The model under review builds one solid part; all positions refer to its coordinate system, in mm. Face numbers are marked on the shaded views. A direction names the side the tool comes from. Give positions to 0.01 mm unless a question says otherwise; leave off trailing zeros. Order: outer loops, then holes, each group sorted by start corner. A loop starts at its lowest first (then second) coordinate and runs counter-clockwise, first axis right, second up. Notation, with made-up numbers: (-20.75, 57.25) -> (-0.75, 57.25) arc R29 cw to (-0.75, 82.25) -> close; hole circle Ø9 at (27, 36.5). An arc over 180 degrees is marked (long way). Use one line per item in the form item = value.
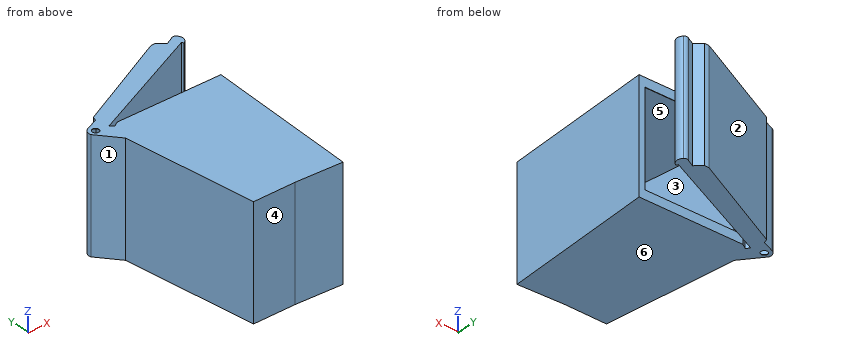
```python
from build123d import *

# Parameters (mm, degrees)
BOSS_EXTRUDE1_DEPTH = 6.35
SHELL1_START        = 0.0254
SHELL1_DEPTH        = 6.2992
SKETCH3_W           = 5.418512696
SKETCH3_H           = 5.334
CUT_EXTRUDE2_DEPTH  = 1.524
SKETCH4_R           = 0.1905
CUT_EXTRUDE3_DEPTH  = 20.633989303


# Read off the part's stored shape, not the designer's step: Shell1
with BuildPart() as part:
    # Sketch1 → Boss-Extrude1 (new body)
    with BuildSketch(Plane.XY):
        with BuildLine():
            Line((7.716040042, 1.833305163), (10.375382868, 1.693751976))
            Line((10.375382868, 1.693751976), (11.029172055, 10.583751976))
            Line((11.029172055, 10.583751976), (5.064666493, 10.656097731))
            Line((5.064666493, 10.656097731), (4.767245057, 10.479252552))
            Line((4.767245057, 10.479252552), (4.590399878, 10.656097731))
            Line((4.590399878, 10.656097731), (11.46006589, 13.704368441))
            Line((11.46006589, 13.704368441), (11.509343406, 13.593315288))
            ThreePointArc((11.509343406, 13.593315288), (11.739536715, 13.882052013), (11.634947175, 14.236197299))
            ThreePointArc((11.634947175, 14.236197299), (11.492158572, 14.298396741), (11.347210136, 14.241411598))
            Line((11.347210136, 14.241411598), (10.931187512, 14.042030874))
            Line((10.931187512, 14.042030874), (10.548202312, 14.393751976))
            Line((10.548202312, 14.393751976), (10.290273504, 14.393751976))
            Line((10.290273504, 14.393751976), (4.530564215, 11.633385245))
            Line((4.530564215, 11.633385245), (4.445957531, 11.39304745))
            Line((4.445957531, 11.39304745), (3.74568803, 11.102479142))
            ThreePointArc((3.74568803, 11.102479142), (3.54655055, 10.911956466), (3.527947792, 10.636986353))
            Line((3.527947792, 10.636986353), (4.481389231, 9.429510304))
            Line((4.481389231, 9.429510304), (5.295382868, 1.833305163))
            Line((5.295382868, 1.833305163), (7.716040042, 1.833305163))
        make_face()
    extrude(amount=BOSS_EXTRUDE1_DEPTH)

    # Shell1 outline → Shell1 (cut)
    with BuildSketch(Plane.XY.offset(SHELL1_START)):
        with BuildLine():
            Line((5.318206472, 1.858705163), (7.716706036, 1.858705163))
            Line((7.716706036, 1.858705163), (10.351875533, 1.720420509))
            Line((10.351875533, 1.720420509), (11.001859717, 10.558681389))
            Line((11.001859717, 10.558681389), (5.071504797, 10.630612918))
            Line((5.071504797, 10.630612918), (4.76325019, 10.447326395))
            Line((4.76325019, 10.447326395), (4.546271575, 10.664305009))
            Line((4.546271575, 10.664305009), (11.472980817, 13.737887461))
            Line((11.472980817, 13.737887461), (11.521908422, 13.627622875))
            ThreePointArc((11.521908422, 13.627622875), (11.716832945, 13.899435369), (11.616664188, 14.218565158))
            ThreePointArc((11.616664188, 14.218565158), (11.489713166, 14.273025818), (11.362015112, 14.220340596))
            Line((11.362015112, 14.220340596), (10.926665769, 14.011697454))
            Line((10.926665769, 14.011697454), (10.538308623, 14.368351976))
            Line((10.538308623, 14.368351976), (10.296045707, 14.368351976))
            Line((10.296045707, 14.368351976), (4.551029407, 11.615026927))
            Line((4.551029407, 11.615026927), (4.466154882, 11.373928288))
            Line((4.466154882, 11.373928288), (3.755422691, 11.079018614))
            ThreePointArc((3.755422691, 11.079018614), (3.570543876, 10.903284548), (3.550847191, 10.64897238))
            Line((3.550847191, 10.64897238), (4.505864047, 9.439501161))
            Line((4.505864047, 9.439501161), (5.318206472, 1.858705163))
        make_face()
    extrude(amount=SHELL1_DEPTH, mode=Mode.SUBTRACT)

    # Sketch3 → Cut-Extrude2 (cut)
    with BuildSketch(Plane(origin=(0.12997786, 10.715952445, 0), x_dir=(0.9999264471855748, -0.012128487903857954, 0), z_dir=(0.012128487903857952, 0.9999264471855747, 0))):
        with Locations((7.850713163, -3.175)):
            Rectangle(SKETCH3_W, SKETCH3_H)
    extrude(amount=-CUT_EXTRUDE2_DEPTH, mode=Mode.SUBTRACT)

    # Sketch4 → Cut-Extrude3 (cut, through all)
    with BuildSketch(Plane.XY.offset(6.35)):
        with Locations((3.89174221, 10.750488628)):
            Circle(SKETCH4_R)
    extrude(amount=-CUT_EXTRUDE3_DEPTH, mode=Mode.SUBTRACT)


solid = part.part
```
1. Add section B-B on y = 3.5. Give the boundary of the cut face in (x, z), then the cut area to 3 significant figures.
Values:
outline = (5.12, 0) -> (10.51, 0) -> (10.51, 6.35) -> (5.12, 6.35) -> close; hole (5.14, 0.03) -> (10.48, 0.03) -> (10.48, 6.32) -> (5.14, 6.32) -> close
area = 0.595 mm^2
2. Tool access review of the marked faces 4, 5 and 6: name each direction out of +Z, -Z, +X, -X, +Y, -Y from which nothing blocks a thin tool from reaching the whole face with its end or side.
Values:
face_4 = +Z, -Z, -X, -Y
face_5 = none
face_6 = -Z, +X, -X, +Y, -Y
3. Add section D-D on y = 10.25. Give the boundary of the cut face in (x, z), then the cut area to 3 significant figures.
Values:
outline = (3.83, 0) -> (11, 0) -> (11, 6.35) -> (3.83, 6.35) -> close; hole (3.87, 0.03) -> (10.98, 0.03) -> (10.98, 6.32) -> (3.87, 6.32) -> close
area = 0.729 mm^2
4. For pin 1 Ø2.5 at (x, z) = (6, 2.5) entering from -Y; pin 2 Ø0.7 at (x, z) = (6.5, 4) entering from +Y (3 decimals); pin 3 Ø1.5 at (x, z) = (7, 5.5) entering from +Y, all flat-tipped, find the tip position at first contact; note any pin that passes through.
Values:
pin_1 = 1.83
pin_2 = 12.745
pin_3 = 13.18
5. The part is to be moulded in two halves that separate along Y. For the marked faces 1, 2 and 3, say which applies: +Y half, -Y half, draft (parallel to the pull), parting line (faces both ways), or undercut.
Values:
face_1 = -Y half
face_2 = +Y half
face_3 = undercut
6. Add section A-A on x = 8.25. Count the separate pieces of the cut face and the enclosed holes in it, then the cut area to 3 significant figures.
Values:
separate_pieces = 2
enclosed_holes = 1
area = 1.04 mm^2
